from build123d import *

# Parameters (mm, degrees)
F0_W      = 70
F0_H      = 35
F1_DEPTH  = 1.5
F2_R      = 4.5
F3_DEPTH  = 12
F4_W      = 8.664048
F4_H      = 7.426328
F5_DEPTH  = 3
F6_W      = 11
F6_H      = 11
F7_DEPTH  = 8
F8_R      = 1
F9_R      = 1
F10_W     = 25
F10_H     = 15
F11_DEPTH = 7
F12_W     = 6
F12_H     = 10
F13_DEPTH = 9
F14_SIZE  = 2
F15_SIZE  = 2


with BuildPart() as f1:
    # F0 (on Top) → F1 (new body)
    with BuildSketch(Plane.XY):
        Rectangle(F0_W, F0_H)
    extrude(amount=-F1_DEPTH)

    # F2 (on Top) → F3 (join)
    with BuildSketch(Plane.XY):
        with Locations((-20, 10)):
            Circle(F2_R)
        with Locations((20, 10)):
            Circle(F2_R)
    extrude(amount=F3_DEPTH)

    # F4 (on Top) → F5 (join)
    with BuildSketch(Plane.XY):
        with Locations((-7.271611, 10.2112)):
            Rectangle(F4_W, F4_H)
    extrude(amount=F5_DEPTH)

    # F6 (on Top) → F7 (join)
    with BuildSketch(Plane.XY):
        with Locations((7.962182, 8.088716)):
            Rectangle(F6_W, F6_H)
    extrude(amount=F7_DEPTH)

    # F8
    f8_edges = [f1.edges().sort_by_distance(p)[0] for p in [
        (13.462182, 13.588716, 4),
    ]]
    fillet(f8_edges, radius=F8_R)

    # F9
    f9_edges = [f1.edges().sort_by_distance(p)[0] for p in [
        (2.462182, 2.588716, 4),
        (13.462182, 2.588716, 4),
        (2.462182, 13.588716, 4),
    ]]
    fillet(f9_edges, radius=F9_R)

    # F10 (on Top) → F11 (join)
    with BuildSketch(Plane.XY):
        with Locations((0.464146, -8.447183)):
            Rectangle(F10_W, F10_H)
    extrude(amount=F11_DEPTH)

    # F12 (on Top) → F13 (join)
    with BuildSketch(Plane.XY):
        with Locations((26.690762, -5)):
            Rectangle(F12_W, F12_H)
        with Locations((-27.694009, -4.952371)):
            Rectangle(F12_W, F12_H)
    extrude(amount=F13_DEPTH)

    # F14
    f14_edges = [f1.edges().sort_by_distance(p)[0] for p in [
        (-24.694009, -4.952371, 9),
    ]]
    chamfer(f14_edges, length=F14_SIZE)

    # F15
    f15_edges = [f1.edges().sort_by_distance(p)[0] for p in [
        (23.690762, -5, 9),
    ]]
    chamfer(f15_edges, length=F15_SIZE)


solid = f1.part
Read the model definition and answer for the solid it produces. Units are mm, in the model's axes. A direction names the side the tool comes from. Give positions to 0.01 mm unless a question says otherwise; leave off trailing zeros. Write each loop counter-clockwise with the first axis right and the second up, starting at its lowest first coordinate (ties: lowest second). Pieces come first, ordered by that corner, then holes. Notation, with made-up numbers: M 17,59 L 21,59 A31 cw 21,87 Z; hole C 12.25,-37 d4. An arc over 180 degrees is marked long. One line per item, written item: value. Start each with the question number.
(1) Find section B-B (y = 10). Determine the outline of the cut face in (x, z), plus the area to 3 significant figures.
(2) Find section A-A (z = 2.25). Determine the outline of the cut face in (x, y).
(3) Find the intervals of material crossed by line 1 (X direction, y = -2.5, z = 1.25); line 2 (Y direction, x = -5, z = 1.75); line 3 (X direction, y = 7.5, z = 7.25), in increasing order.
(4) Determine the mould class of faces 1 (the flat face through (-28, -9.952, 4)), 2 (the flat face through (-11.604, 10, 1)), 3 (the flat face through (-35, 0, -1)) for opening direction X: pulls with the +X half, pulls with the -X half, needs draft (parallel to the pull), parting line crosses it, or undercut.
(5) Find section D-D (x = -20). Determine the outline of the cut face in (y, z).
(6) A tool of negligible diameter and unlimited length cuts with its end or side. For faces 4 (the cylindrical face through (15.504, 10.198, 5.916)), 5 (the flat face through (-2.94, 10, 1)), 6 (the flat face through (8, 2.589, 4)), 7 (the flat face through (-24.694, -5, 3)), 8 (the flat face through (24.7, -5.07, 8.01)), from which of +Z, -Z, +X, -X, +Y, -Y can it reach the whole face along a straight path? Write none if from no direction.
(7) Find section C-C (x = -29). Determine the outline of the cut face in (y, z), plus the area to 4 significant figures.
(8) Flat-ended cylindrical pins translate along their axes: pin 1 Ø6.5 at (y, z) = (9.5, 4) entering from +X; pin 2 Ø2.5 at (y, z) = (9, 1.5) entering from -X; pin 3 Ø1.5 at (y, z) = (11.5, 5) entering from -X. Find the tip coordinate at first contact, or state that the pin passes through.
Results below:
1. outline: M -35,-1.5 L 35,-1.5 L 35,0 L 24.5,0 L 24.5,12 L 15.5,12 L 15.5,0 L 13.46,0 L 13.46,8 L 2.46,8 L 2.46,0 L -2.94,0 L -2.94,3 L -11.6,3 L -11.6,0 L -15.5,0 L -15.5,12 L -24.5,12 L -24.5,0 L -35,0 Z
1. area: 435 mm^2
2. outline: M -30.69,-9.95 L -24.69,-9.95 L -24.69,0.05 L -30.69,0.05 Z; C -20,10 d9; M -12.04,-15.95 L 12.96,-15.95 L 12.96,-0.95 L -12.04,-0.95 Z; M -11.6,6.5 L -2.94,6.5 L -2.94,13.92 L -11.6,13.92 Z; M 2.46,3.59 A1 ccw 3.46,2.59 L 12.46,2.59 A1 ccw 13.46,3.59 L 13.46,12.59 A1 ccw 12.46,13.59 L 3.46,13.59 A1 ccw 2.46,12.59 Z; C 20,10 d9; M 23.69,-10 L 29.69,-10 L 29.69,0 L 23.69,0 Z
3. line 1: x = -30.69 to -24.69, -12.04 to 12.96, 23.69 to 29.69
3. line 2: y = -15.95 to -0.95, 6.5 to 13.92
3. line 3: x = -23.74 to -16.26, 2.46 to 13.46, 16.26 to 23.74
4. face 1: needs draft
4. face 2: undercut
4. face 3: pulls with the -X half
5. outline: M -17.5,-1.5 L 17.5,-1.5 L 17.5,0 L 14.5,0 L 14.5,12 L 5.5,12 L 5.5,0 L -17.5,0 Z
6. face 4: +Z
6. face 5: +Z, +Y
6. face 6: +Z, +X, -X
6. face 7: +Z, +Y, -Y
6. face 8: +Z, -Y
7. outline: M -17.5,-1.5 L 17.5,-1.5 L 17.5,0 L 0.05,0 L 0.05,9 L -9.95,9 L -9.95,0 L -17.5,0 Z
7. area: 142.5 mm^2
8. pin 1: stops at x = 24.5
8. pin 2: stops at x = -24.5
8. pin 3: stops at x = -24.44
